Can you work these out from the model? Positions are in its coordinate system, mm. Round coordinates to 2 decimals unless told otherwise and drop trailing zeros. Order: outer loops, then holes, each group sorted by start corner. A loop starts at its lowest first (then second) coordinate and runs counter-clockwise, first axis right, second up. Notation, with made-up numbers: (-24.75, 43.25) -> (28.25, 43.25) arc R22 ccw to (28.25, 56.25) -> close; hole circle Ø5 at (68, 49.25). An arc over 180 degrees is marked (long way). Use a Markdown table: item, result. Add a question column.
Q1. If we section it at A-A on z = 4: List the corners of the cut face in (x, y) for me, plus the area to 3 significant figures.
Q2. I need wall thicknesses on line 1 along Z through (x, y) = (28, 5.5); line 2 along Y through (x, z) = (-20, -15.5); line 3 along X through (y, z) = (2.5, 13). Which ranges of each line are inside material? Lowest first, please. Write a range as [from, to].
Q3. If we section it at C-C on x = -18: List the corners of the cut face in (y, z) for me, plus the area to 3 significant figures.
Q4. I'm going to push flat-ended pins straight in: pin 1 Ø1.5 at (x, z) = (17, -6.5) entering from +Y; pin 2 Ø6 at (y, z) = (15, 1.5) entering from -X; pin 3 Ø12 at (y, z) = (-22, 14) entering from -X. Where does each tip first touch, or does it pass through?
Q5. We'd pull the mould along X, two halves only. Please class faces 1 (the face through (-12, 29, -22)), 2 (the face through (0, 0, -2)), 3 (the face through (0, 0, 0)): +X half, -X half, draft (parallel to the pull), parting line (faces both ways), or undercut.
Q6. If we section it at B-B on y = 11: List the corners of the cut face in (x, z) for me, plus the area to 3 significant figures.
```python
from build123d import *

# Parameters (mm, degrees)
F1_DEPTH = 20
F2_DEPTH = 22
F3_DEPTH = 2


with BuildPart() as f1:
    # F0 (on Top) → F1 (new body)
    with BuildSketch(Plane.XY):
        with BuildLine():
            ThreePointArc((0, -32), (22.627417, -22.627417), (32, 0))
            ThreePointArc((32, 0), (22.627417, 22.627417), (0, 32))
            Line((0, 32), (0, 31))
            ThreePointArc((0, 31), (21.92031, 21.92031), (31, 0))
            ThreePointArc((31, 0), (21.92031, -21.92031), (0, -31))
            Line((0, -31), (0, -32))
        make_face()
        with BuildLine():
            Line((0, 31), (0, 32))
            ThreePointArc((0, 32), (-32, 0), (0, -32))
            Line((0, -32), (0, -31))
            ThreePointArc((0, -31), (-31, 0), (0, 31))
        make_face()
    extrude(amount=F1_DEPTH)

    # F0 (on Top) → F2 (join)
    with BuildSketch(Plane.XY):
        with BuildLine():
            ThreePointArc((0, -32), (22.627417, -22.627417), (32, 0))
            ThreePointArc((32, 0), (22.627417, 22.627417), (0, 32))
            Line((0, 32), (0, 31))
            ThreePointArc((0, 31), (21.92031, 21.92031), (31, 0))
            ThreePointArc((31, 0), (21.92031, -21.92031), (0, -31))
            Line((0, -31), (0, -32))
        make_face()
        with BuildLine():
            Line((0, 31), (0, 32))
            ThreePointArc((0, 32), (-32, 0), (0, -32))
            Line((0, -32), (0, -31))
            ThreePointArc((0, -31), (-31, 0), (0, 31))
        make_face()
    extrude(amount=-F2_DEPTH)

    # F0 (on Top) → F3 (join)
    with BuildSketch(Plane.XY):
        with BuildLine():
            ThreePointArc((31, 0), (21.92031, 21.92031), (0, 31))
            Line((0, 31), (0, -31))
            ThreePointArc((0, -31), (21.92031, -21.92031), (31, 0))
        make_face()
        with BuildLine():
            Line((0, -31), (0, 31))
            ThreePointArc((0, 31), (-31, 0), (0, -31))
        make_face()
        with BuildLine():
            Line((0, 31), (0, 32))
            ThreePointArc((0, 32), (-32, 0), (0, -32))
            Line((0, -32), (0, -31))
            ThreePointArc((0, -31), (-31, 0), (0, 31))
        make_face()
        with BuildLine():
            ThreePointArc((0, -32), (22.627417, -22.627417), (32, 0))
            ThreePointArc((32, 0), (22.627417, 22.627417), (0, 32))
            Line((0, 32), (0, 31))
            ThreePointArc((0, 31), (21.92031, 21.92031), (31, 0))
            ThreePointArc((31, 0), (21.92031, -21.92031), (0, -31))
            Line((0, -31), (0, -32))
        make_face()
    extrude(amount=-F3_DEPTH)


solid = f1.part
```
Answer below:
| question | item | result |
|---|---|---|
| 1 | outline | circle Ø64 at (0, 0); hole (0, 31) arc R31 ccw (long way) to (31, 0) arc R31 ccw to start |
| 1 | area | 198 mm² |
| 2 | line 1 | [-2, 0] |
| 2 | line 2 | [-24.98, -23.69], [23.69, 24.98] |
| 2 | line 3 | [-31.9, -30.9], [30.9, 31.9] |
| 3 | outline | (-26.46, -22) -> (-25.24, -22) -> (-25.24, -2) -> (25.24, -2) -> (25.24, -22) -> (26.46, -22) -> (26.46, 20) -> (25.24, 20) -> (25.24, 0) -> (-25.24, 0) -> (-25.24, 20) -> (-26.46, 20) -> close |
| 3 | area | 203 mm² |
| 4 | pin 1 | y = 27.57 |
| 4 | pin 2 | x = -29.66 |
| 4 | pin 3 | x = -27.71 |
| 5 | face 1 | draft |
| 5 | face 2 | undercut |
| 5 | face 3 | undercut |
| 6 | outline | (-30.05, -22) -> (-28.98, -22) -> (-28.98, -2) -> (28.98, -2) -> (28.98, -22) -> (30.05, -22) -> (30.05, 20) -> (28.98, 20) -> (28.98, 0) -> (-28.98, 0) -> (-28.98, 20) -> (-30.05, 20) -> close |
| 6 | area | 206 mm² |
